The listing builds one solid part. Answer for the finished solid, in the listing's coordinates (mm). A direction names the side the tool comes from. Give positions to 0.01 mm unless a question says otherwise; leave off trailing zeros. Order: outer loops, then holes, each group sorted by start corner. A loop starts at its lowest first (then second) coordinate and runs counter-clockwise, first axis right, second up. Notation, with made-up numbers: (-3, 25.25) -> (45, 25.25) arc R10 ccw to (45, 35.25) -> close; hole circle Ø10 at (72, -32). An arc over 180 degrees is marked (long way). One line per question, with ' | ' between items. Start each with the question number.
```python
from build123d import *

# Parameters (mm, degrees)
F3_DEPTH = 7
F4_D     = 6.7564
F5_COUNT = 4


with BuildPart() as f3:
    # F1 (on Top) → F3 (new body)
    with BuildSketch(Plane.XY):
        with BuildLine():
            Line((-28.5, 12.7), (-40.7, 12.7))
            ThreePointArc((-40.7, 12.7), (-53.4, 0), (-40.7, -12.7))
            Line((-40.7, -12.7), (-28.5, -12.7))
            Line((-28.5, -12.7), (-12.7, -12.7))
            Line((-12.7, -12.7), (0, 0))
            Line((0, 0), (-12.7, 12.7))
            Line((-12.7, 12.7), (-28.5, 12.7))
        make_face()
    extrude(amount=F3_DEPTH)

    # F4 (through all)
    with Locations(Plane(origin=(0, 0, 0), x_dir=(1, 0, 0), z_dir=(0, 0, -1))):
        with Locations((-40.7, 0), (-19.7, 0)):
            Hole(F4_D / 2)

    # F5: F3 ×4 about axis
    f5_axis = Axis((0, 0, 15.328399837), (0, 0, 1))


with BuildPart() as f3_1:
    add(f3.part)
    for i in range(1, F5_COUNT):
        add(f3.part.rotate(f5_axis, i * 360 / F5_COUNT))


solid = f3_1.part
```
(1) The part is cut by section B-B on z = 2. State how many separate pieces and enclosed holes the cut face has, plus the area to 3 significant figures.
(2) Consider line 1 (X direction, y = -40.7, z = 5.75); line 2 (Y direction, x = -2.5, z = 3.75). Determine where each line is inside the solid, lowest interval first.
(3) Determine the mould class of faces 1 (the face through (27, -12.7, 3)), 2 (the face through (-53.397, 0.279, 3.451)), 3 (the face through (43.922, 1.015, 3.549)) for opening direction X: pulls with the +X half, pulls with the -X half, needs draft (parallel to the pull), parting line crosses it, or undercut.
(4) Given P1, Ø6, axis at x = 0, y = 40.7, coming from the -Z side; P2, Ø8, axis at x = 20.5, y = 0.5, coming from the +Z side; P3, Ø2, axis at y = 26.5, z = 2.5, coming from the +X side; P4, Ø3, axis at x = -28.5, z = 2, coming from the -Y side, each flat-ended and moving along its own axis, determine where each tip first touches the part or whether it passes through.
(5) For faces 4 (the face through (-27, 12.7, 3)), 5 (the face through (12.7, 27, 3)), 6 (the face through (-27, -12.7, 3)), determine the directions among +Z, -Z, +X, -X, +Y, -Y from which every point of the face is accessible in a straight line to the end or side of a thin tool.
(6) The part is cut by section C-C on y = 19.7. Determine the outline of the cut face in (x, z).
(7) The part is cut by section A-A on x = 0. Determine the outline of the cut face in (y, z).
Result sheet:
1) separate pieces: 1 | enclosed holes: 8 | area: 4,220 mm^2
2) line 1: x = -12.7 to -3.38, 3.38 to 12.7 | line 2: y = -53.15 to -42.97, -38.43 to -21.97, -17.43 to 17.43, 21.97 to 38.43, 42.97 to 53.15
3) face 1: needs draft | face 2: pulls with the -X half | face 3: undercut
4) P1: passes through | P2: stops at z = 7 | P3: stops at x = 12.7 | P4: stops at y = -12.7
5) face 4: +Z, -Z, -X, +Y | face 5: +Z, -Z, +X, +Y | face 6: +Z, -Z, -X, -Y
6) outline: (-12.7, 0) -> (-3.38, 0) -> (-3.38, 7) -> (-12.7, 7) -> close; (3.38, 0) -> (12.7, 0) -> (12.7, 7) -> (3.38, 7) -> close
7) outline: (-53.4, 0) -> (-44.08, 0) -> (-44.08, 7) -> (-53.4, 7) -> close; (-37.32, 0) -> (-23.08, 0) -> (-23.08, 7) -> (-37.32, 7) -> close; (-16.32, 0) -> (16.32, 0) -> (16.32, 7) -> (-16.32, 7) -> close; (23.08, 0) -> (37.32, 0) -> (37.32, 7) -> (23.08, 7) -> close; (44.08, 0) -> (53.4, 0) -> (53.4, 7) -> (44.08, 7) -> close
